Design review of the part built by this model. Coordinates are the model's own, in mm. Coordinates: 2 decimals unless noted, no trailing zeros. Order: outer loops, then holes, each group sorted by start corner. A loop starts at its lowest first (then second) coordinate and runs counter-clockwise, first axis right, second up. Notation, with made-up numbers: M 66.25,39.5 L 71.25,39.5 A35 cw 71.25,75.5 Z; hole C 61,38.5 d3. An arc over 180 degrees is marked long. Answer in a Markdown table with one row per item.
from build123d import *

# Parameters (mm, degrees)
MODEL_W                 = 8.2
MODEL_H                 = 3
SALIENTE_EXTRUIR1_DEPTH = 0.1


with BuildPart() as part:
    # Model → Saliente-Extruir1 (new body)
    with BuildSketch(Plane.XY):
        Polygon((50.124922154, 24.617645317), (50.124922154, 19.617645317), (50.887641035, -3.103510086), (34.169357615, -3.381657238), (30.626179611, 10.250358005), (27.083001606, -3.381657238), (10.364718187, -3.103510086), (11.040374185, 25.978480921), (14.626179611, 25.917645317), (14.626179611, 20.295679334), (46.626179611, 20.295679334), (46.626179611, 25.917645317), (50.124922154, 25.9284032), align=None)
        with Locations((18.126179611, 14.017645317)):
            Rectangle(MODEL_W, MODEL_H, mode=Mode.SUBTRACT)
        with Locations((43.126179611, 14.017645317)):
            Rectangle(MODEL_W, MODEL_H, mode=Mode.SUBTRACT)
    extrude(amount=SALIENTE_EXTRUIR1_DEPTH)


solid = part.part
(1) Add section C-C, the plane x = 45. Give the boundary of the cut face in (y, z).
Return value:
| item | result |
|---|---|
| outline | M -3.2,0 L 12.52,0 L 12.52,0.1 L -3.2,0.1 Z; M 15.52,0 L 20.3,0 L 20.3,0.1 L 15.52,0.1 Z |
(2) Add section B-B, the plane y = 1.75. Give the boundary of the cut face in (x, z), and give its area (3 significant figures).
Return value:
| item | result |
|---|---|
| outline | M 10.48,0 L 28.42,0 L 28.42,0.1 L 10.48,0.1 Z; M 32.84,0 L 50.72,0 L 50.72,0.1 L 32.84,0.1 Z |
| area | 3.58 mm2 |
(3) Add section D-D, the plane x = 23.5. Give the boundary of the cut face in (y, z), and give its area (3 significant figures).
Return value:
| item | result |
|---|---|
| outline | M -3.32,0 L 20.3,0 L 20.3,0.1 L -3.32,0.1 Z |
| area | 2.36 mm2 |
(4) Add section A-A, the plane z = 0.05. Give the boundary of the cut face in (x, y), and give its area (3 significant figures).
Return value:
| item | result |
|---|---|
| outline | M 10.36,-3.1 L 27.08,-3.38 L 30.63,10.25 L 34.17,-3.38 L 50.89,-3.1 L 50.12,19.62 L 50.12,25.93 L 46.63,25.92 L 46.63,20.3 L 14.63,20.3 L 14.63,25.92 L 11.04,25.98 Z; hole M 14.03,12.52 L 22.23,12.52 L 22.23,15.52 L 14.03,15.52 Z; hole M 39.03,12.52 L 47.23,12.52 L 47.23,15.52 L 39.03,15.52 Z |
| area | 882 mm2 |
(5) For line 1 along X through (y, z) = (13, 0.05); line 2 along Y through (x, z) = (46, 0.05); line 3 along X through (y, z) = (21.5, 0.05), list the stretches that pass through material, from the lowest coordinate up. Write a range as from..to.
Return value:
| item | result |
|---|---|
| line 1 | x = 10.74..14.03, 22.23..39.03, 47.23..50.35 |
| line 2 | y = -3.18..12.52, 15.52..20.3 |
| line 3 | x = 10.94..14.63, 46.63..50.12 |
